Can you work these out from the drawing? Everything is in mm from the part's minimum corner. A direction names the side the tool comes from. Round coordinates to 2 decimals unless told otherwise and drop trailing zeros. Loops run counter-clockwise (first coordinate to the right, second up) from the corner with the lowest first, then second, coordinate; pieces in that order, holes last. Notation, with made-up numbers: M -39.75,32.5 L 7.25,32.5 A20 cw 7.25,47.5 Z; hole C 30.25,43.5 d4. An arc over 180 degrees is marked long. Use a Markdown table: item, result.
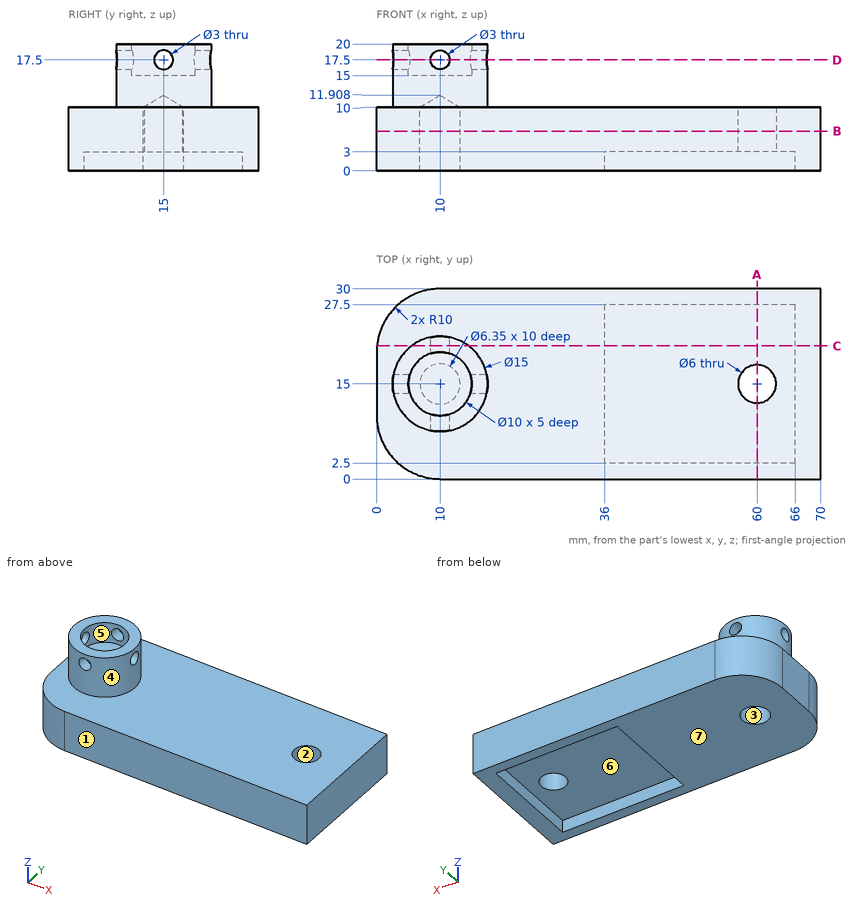
1. I need wall thicknesses on probe 1 along Z at (x, y) = (10, 9); probe 2 along Y at (x, z) = (10, 7.75) (1 decimal); probe 3 along X at (y, z) = (14.25, 5.5) (1 decimal). Which ranges of each line are inside material? Lowest first, please. Write a range as from..to.
Answer sheet:
| item | result |
|---|---|
| probe 1 | 0..16, 19..20 |
| probe 2 | 0..11.8, 18.2..30 |
| probe 3 | 0..6.9, 13.1..57.1, 62.9..70 |
2. Which directions (+Z, -Z, +X, -X, +Y, -Y) give clear straight access to the entire face, cutting with the end or side of a thin tool? Please do the marked faces 5, 6 and 7.
Answer sheet:
| item | result |
|---|---|
| face 5 | +Z |
| face 6 | -Z |
| face 7 | -Z, +X, -X, +Y, -Y |
3. Imagine slicing it at C-C, the plane y = 21. Write out the boundary of the cut face in (x, z).
Answer sheet:
| item | result |
|---|---|
| outline | M 0.05,0 L 36,0 L 36,3 L 66,3 L 66,0 L 70,0 L 70,10 L 14.5,10 L 14.5,20 L 5.5,20 L 5.5,10 L 0.05,10 Z; hole C 10,17.5 d3 |
4. We'd pull the mould along X, two halves only. Please class the marked faces 1, 2, 3 and 4: +X half, -X half, draft (parallel to the pull), parting line (faces both ways), or undercut.
Answer sheet:
| item | result |
|---|---|
| face 1 | draft |
| face 2 | undercut |
| face 3 | undercut |
| face 4 | parting line |
5. Imagine slicing it at A-A, the plane x = 60. Write out the boundary of the cut face in (y, z), then the cut area to 3 significant figures.
Answer sheet:
| item | result |
|---|---|
| outline | M 0,0 L 2.5,0 L 2.5,3 L 12,3 L 12,10 L 0,10 Z; M 18,3 L 27.5,3 L 27.5,0 L 30,0 L 30,10 L 18,10 Z |
| area | 183 mm2 |
6. Imagine slicing it at B-B, the plane z = 6.25. State how many separate pieces and enclosed holes the cut face has, then the cut area to 3 significant figures.
Answer sheet:
| item | result |
|---|---|
| separate pieces | 1 |
| enclosed holes | 2 |
| area | 2,000 mm2 |
7. For pin 1 Ø4 at (y, z) = (15, 17.5) entering from -X; pin 2 Ø10 at (x, y) = (47.5, 12) entering from -Z; pin 3 Ø15 at (x, y) = (32.5, 11.5) entering from +Z, each with a flat end and sliding along its axis, tell me the tip position at first contact or that it passes through.
Answer sheet:
| item | result |
|---|---|
| pin 1 | x = 2.5 |
| pin 2 | z = 3 |
| pin 3 | z = 10 |
8. Imagine slicing it at D-D, the plane z = 17.5. Write out the boundary of the cut face in (x, y).
Answer sheet:
| item | result |
|---|---|
| outline | M 2.65,13.5 A7.5 ccw 8.5,7.65 L 8.5,10.23 A5 cw 5.23,13.5 Z; M 2.65,16.5 L 5.23,16.5 A5 cw 8.5,19.77 L 8.5,22.35 A7.5 ccw Z; M 11.5,7.65 A7.5 ccw 17.35,13.5 L 14.77,13.5 A5 cw 11.5,10.23 Z; M 11.5,19.77 A5 cw 14.77,16.5 L 17.35,16.5 A7.5 ccw 11.5,22.35 Z |
